```python
from build123d import *

# Parameters (mm, degrees)
SKETCH1_R           = 12.7
SKETCH1_R_2         = 3.175
BOSS_EXTRUDE1_DEPTH = 10
SKETCH1_3_R         = 12.7
SKETCH1_3_R_2       = 6.35
BOSS_EXTRUDE2_DEPTH = 2.5
SKETCH2_R           = 12.7
BOSS_EXTRUDE3_DEPTH = 10
SKETCH3_R           = 5
CUT_EXTRUDE3_DEPTH  = 10
CUT_EXTRUDE4_START  = -1.45
SKETCH4_R           = 10
CUT_EXTRUDE4_DEPTH  = 5
CUT_EXTRUDE5_DEPTH  = 2
SKETCH7_R           = 10
CUT_EXTRUDE7_DEPTH  = 6.45
BOSS_EXTRUDE4_START = 6.45
SKETCH8_R           = 10
SKETCH8_R_2         = 9.5625
BOSS_EXTRUDE4_DEPTH = 6.45
BOSS_EXTRUDE5_START = -8
BOSS_EXTRUDE5_DEPTH = 8
FILLET1_R           = 2.5


with BuildPart() as part:
    # Sketch1 → Boss-Extrude1 (new body)
    with BuildSketch(Plane(origin=(0, 0, 0), x_dir=(1, 0, 0), z_dir=(0, 1, 0))):
        with BuildLine():
            Line((-41.199040767, 52.757793765), (38.800959233, 52.757793765))
            ThreePointArc((38.800959233, 52.757793765), (45.872027044, 49.828861577), (48.800959233, 42.757793765))
            Line((48.800959233, 42.757793765), (48.800959233, -37.242206235))
            ThreePointArc((48.800959233, -37.242206235), (45.872027044, -44.313274047), (38.800959233, -47.242206235))
            Line((38.800959233, -47.242206235), (-41.199040767, -47.242206235))
            ThreePointArc((-41.199040767, -47.242206235), (-48.270108579, -44.313274047), (-51.199040767, -37.242206235))
            Line((-51.199040767, -37.242206235), (-51.199040767, 42.757793765))
            ThreePointArc((-51.199040767, 42.757793765), (-48.270108579, 49.828861577), (-41.199040767, 52.757793765))
        make_face()
        with Locations(Location((0, 0, 0), (0, 0, 270))):
            Circle(SKETCH1_R, mode=Mode.SUBTRACT)
        with Locations(Location((-41.199040767, 42.757793765, 0), (0, 0, 270))):
            Circle(SKETCH1_R_2, mode=Mode.SUBTRACT)
        with Locations(Location((38.800959233, 42.757793765, 0), (0, 0, 270))):
            Circle(SKETCH1_R_2, mode=Mode.SUBTRACT)
        with Locations(Location((38.800959233, -37.242206235, 0), (0, 0, 270))):
            Circle(SKETCH1_R_2, mode=Mode.SUBTRACT)
        with Locations(Location((-41.199040767, -37.242206235, 0), (0, 0, 270))):
            Circle(SKETCH1_R_2, mode=Mode.SUBTRACT)
    extrude(amount=BOSS_EXTRUDE1_DEPTH)

    # Sketch1<3> → Boss-Extrude2 (add)
    with BuildSketch(Plane(origin=(0, 0, 0), x_dir=(1, 0, 0), z_dir=(0, 1, 0))):
        with Locations(Location((0, 0, 0), (0, 0, 270))):
            Circle(SKETCH1_3_R)
        with Locations(Location((0, 0, 0), (0, 0, 270))):
            Circle(SKETCH1_3_R_2, mode=Mode.SUBTRACT)
    extrude(amount=BOSS_EXTRUDE2_DEPTH)

    # Sketch2 → Boss-Extrude3 (add, through all)
    with BuildSketch(Plane(origin=(0, 10, 0), x_dir=(1, 0, 0), z_dir=(0, 1, 0))):
        Circle(SKETCH2_R)
    extrude(amount=-BOSS_EXTRUDE3_DEPTH)

    # Sketch3 → Cut-Extrude3 (cut)
    with BuildSketch(Plane(origin=(0, 10, 0), x_dir=(1, 0, 0), z_dir=(0, 1, 0))):
        with Locations(Location((-1.199040767, 2.757793765, 0), (0, 0, 270))):
            Circle(SKETCH3_R)
    extrude(amount=-CUT_EXTRUDE3_DEPTH, mode=Mode.SUBTRACT)

    # Sketch4 → Cut-Extrude4 (cut)
    with BuildSketch(Plane(origin=(0, 10, 0), x_dir=(1, 0, 0), z_dir=(0, 1, 0)).offset(CUT_EXTRUDE4_START)):
        with Locations(Location((-1.199040767, 2.757793765, 0), (0, 0, 270))):
            Circle(SKETCH4_R)
    extrude(amount=-CUT_EXTRUDE4_DEPTH, mode=Mode.SUBTRACT)

    # Sketch6 → Cut-Extrude5 (cut)
    with BuildSketch(Plane.XZ):
        with BuildLine():
            Line((48.800959233, -42.757793765), (48.800959233, 37.242206235))
            ThreePointArc((48.800959233, 37.242206235), (45.872027044, 44.313274047), (38.800959233, 47.242206235))
            Line((38.800959233, 47.242206235), (-41.199040767, 47.242206235))
            ThreePointArc((-41.199040767, 47.242206235), (-48.270108579, 44.313274047), (-51.199040767, 37.242206235))
            Line((-51.199040767, 37.242206235), (-51.199040767, -42.757793765))
            ThreePointArc((-51.199040767, -42.757793765), (-48.270108579, -49.828861577), (-41.199040767, -52.757793765))
            Line((-41.199040767, -52.757793765), (38.800959233, -52.757793765))
            ThreePointArc((38.800959233, -52.757793765), (45.872027044, -49.828861577), (48.800959233, -42.757793765))
        make_face()
    extrude(amount=-CUT_EXTRUDE5_DEPTH, mode=Mode.SUBTRACT)

    # Sketch7 → Cut-Extrude7 (cut)
    with BuildSketch(Plane(origin=(0, 10, 0), x_dir=(1, 0, 0), z_dir=(0, 1, 0))):
        with Locations(Location((-1.199040767, 2.757793765, 0), (0, 0, 270))):
            Circle(SKETCH7_R)
    extrude(amount=-CUT_EXTRUDE7_DEPTH, mode=Mode.SUBTRACT)

    # Sketch8 → Boss-Extrude4 (add)
    with BuildSketch(Plane(origin=(0, 3.55, 0), x_dir=(1, 0, 0), z_dir=(0, 1, 0)).offset(BOSS_EXTRUDE4_START)):
        with Locations((-1.199040767, 2.757793765)):
            Circle(SKETCH8_R)
        with Locations(Location((-1.199040767, 2.757793765, 0), (0, 0, 270))):
            Circle(SKETCH8_R_2, mode=Mode.SUBTRACT)
    extrude(amount=-BOSS_EXTRUDE4_DEPTH)

    # Sketch9 → Boss-Extrude5 (add)
    with BuildSketch(Plane(origin=(0, 10, 0), x_dir=(1, 0, 0), z_dir=(0, 1, 0)).offset(BOSS_EXTRUDE5_START)):
        with BuildLine():
            Line((-51.199040767, 42.757793765), (-51.199040767, 52.757793765))
            Line((-51.199040767, 52.757793765), (-41.199040767, 52.757793765))
            ThreePointArc((-41.199040767, 52.757793765), (-48.270108579, 49.828861577), (-51.199040767, 42.757793765))
        make_face()
        with BuildLine():
            Line((38.800959233, 52.757793765), (48.800959233, 52.757793765))
            Line((48.800959233, 52.757793765), (48.800959233, 42.757793765))
            ThreePointArc((48.800959233, 42.757793765), (45.872027044, 49.828861577), (38.800959233, 52.757793765))
        make_face()
        with BuildLine():
            Line((-51.199040767, -37.242206235), (-51.199040767, -47.242206235))
            Line((-51.199040767, -47.242206235), (-41.199040767, -47.242206235))
            ThreePointArc((-41.199040767, -47.242206235), (-48.270108579, -44.313274047), (-51.199040767, -37.242206235))
        make_face()
        with BuildLine():
            Line((48.800959233, -37.242206235), (48.800959233, -47.242206235))
            Line((48.800959233, -47.242206235), (38.800959233, -47.242206235))
            ThreePointArc((38.800959233, -47.242206235), (45.872027044, -44.313274047), (48.800959233, -37.242206235))
        make_face()
    extrude(amount=BOSS_EXTRUDE5_DEPTH)

    # Fillet1
    fillet1_edges = [part.edges().sort_by_distance(p)[0] for p in [
        (-51.199040767, 6, -52.757793765),
        (48.800959233, 6, -52.757793765),
        (48.800959233, 6, 47.242206235),
        (-51.199040767, 6, 47.242206235),
    ]]
    fillet(fillet1_edges, radius=FILLET1_R)


solid = part.part
```
Could you check a few things on this model? Use its own coordinates, in mm. A direction names the side the tool comes from. Give positions to 0.01 mm unless a question says otherwise; leave off trailing zeros. Write each loop counter-clockwise with the first axis right and the second up, starting at its lowest first coordinate (ties: lowest second). Pieces come first, ordered by that corner, then holes. Notation, with made-up numbers: (-4.5, -19.75) - (13.5, -19.75) arc R8 ccw to (13.5, -8.75) - close; hole circle Ø8 at (4.25, 66). An arc over 180 degrees is marked (long way). One line per item, written item: value. Start each with the question number.
Item 1: I'm going to push flat-ended pins straight in: pin 1 (22 mm diameter, centred on x = -1.2, z = -2.76, fed in from +Y); pin 2 (5.5 mm diameter, centred on x = 38.8, z = -42.76, fed in from -Y). Where does each tip first touch, or does it pass through?
Item 2: Which directions (+Z, -Z, +X, -X, +Y, -Y) give clear straight access to the entire face, cutting with the end or side of a thin tool? Please do faces 4 (the face through (-5, 3.55, 1)), 5 (the face through (-44.016, 5.944, 38.707)).
Item 3: Imagine slicing it at A-A, the plane z = -0.5. List the corners of the cut face in (x, y) for me.
Item 4: Please list where these lines run through material, in increasing order: line 1 (Z direction, x = -41.5, y = 4.75); line 2 (Z direction, x = 37, y = 3); line 3 (X direction, y = 9.5, z = -4). Write a range as from..to.
Item 5: If we mould it in two halves opening along Z, with no side actions, what happens to faces 1 (the face through (-50.486, 6.056, -52.006)), 2 (the face through (-4.241, 2.786, -6.726)), 3 (the face through (-1, 6, 47.242))? For each: +Z half, -Z half, draft (parallel to the pull), parting line (faces both ways), or undercut.
Item 6: Imagine slicing it at B-B, the plane y = 8.5. Give the number of separate pieces and of enclosed holes in the cut face, and give its area (3 significant figures).
Geometry says:
1. pin 1: y = 10
1. pin 2: through
2. face 4: +Y
2. face 5: +Y, -Y
3. outline: (-51.2, 2) - (-5.66, 2) - (-5.66, 3.55) - (-10.49, 3.55) - (-10.49, 10) - (-51.2, 10) - close; (3.26, 2) - (48.8, 2) - (48.8, 10) - (8.09, 10) - (8.09, 3.55) - (3.26, 3.55) - close
4. line 1: -52.76..-45.92, -39.6..34.08, 40.4..47.24
4. line 2: -52.76..-45.37, -40.14..34.63, 39.86..47.24
4. line 3: -51.2..-10.68, 8.28..48.8
5. face 1: -Z half
5. face 2: undercut
5. face 3: +Z half
6. separate pieces: 1
6. enclosed holes: 5
6. area: 9,580 mm^2
